Can you work these out from the drawing? Everything is in mm from the part's minimum corner. A direction names the side the tool comes from. Coordinates: 2 decimals unless noted, no trailing zeros. Write each loop counter-clockwise with the first axis right and the second up, starting at its lowest first coordinate (ties: lowest second). Pieces come first, ordered by that corner, then holes. Notation, with made-up numbers: M 86.5,29 L 133.5,29 A14 ccw 133.5,45 Z; hole C -28,30.5 d4. An arc over 180 degrees is marked long. Write item = value, one per line.
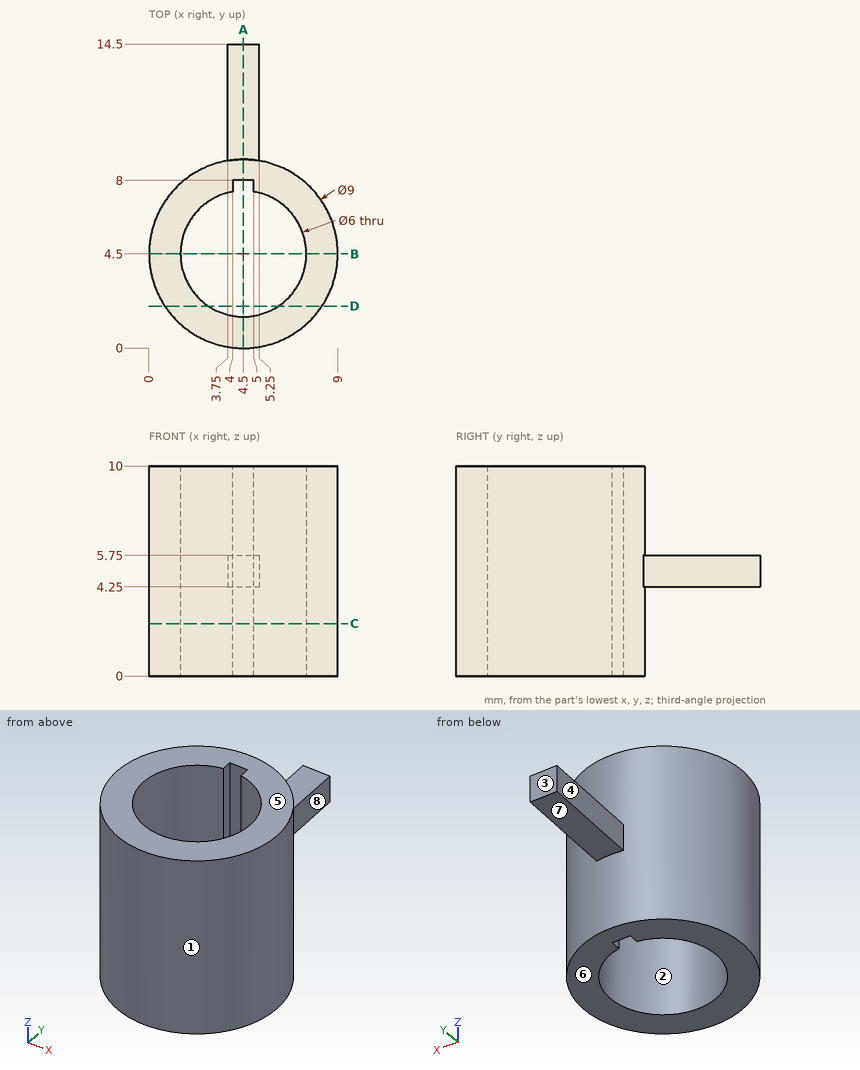
Item 1: For the marked faces 4, 5, 6, 7 and 8, which set-ups out of +Z, -Z, +X, -X, +Y, -Y let a thin tool reach every point of the face, with its end or its side?
Numbers:
face_4 = +Z, -Z, -X, +Y
face_5 = +Z, +X, -X, +Y, -Y
face_6 = -Z, +X, -X, +Y, -Y
face_7 = -Z, +X, -X, +Y
face_8 = +Z, -Z, +X, +Y
Item 2: I'm going to push flat-ended pins straight in: P1, Ø1, axis at y = 10, z = 5, coming from the +X side; P2, Ø1.6, axis at x = 4.5, y = 11.5, coming from the +Z side; P3, Ø6, axis at y = 12, z = 4.5, coming from the -X side. Where does each tip first touch, or does it pass through?
Numbers:
P1 = 5.25
P2 = 5.75
P3 = 3.75
Item 3: Imagine slicing it at D-D (y = 2). Write out the boundary of the cut face in (x, z).
Numbers:
outline = M 0.76,0 L 2.84,0 L 2.84,10 L 0.76,10 Z; M 6.16,0 L 8.24,0 L 8.24,10 L 6.16,10 Z
Item 4: Imagine slicing it at C-C (z = 2.5). Write out the boundary of the cut face in (x, y).
Numbers:
outline = C 4.5,4.5 d9; hole M 4,7.46 A3 ccw long 5,7.46 L 5,8 L 4,8 Z
Item 5: Imagine slicing it at B-B (y = 4.5). Write out the boundary of the cut face in (x, z), and give its area (3 significant figures).
Numbers:
outline = M 0,0 L 1.5,0 L 1.5,10 L 0,10 Z; M 7.5,0 L 9,0 L 9,10 L 7.5,10 Z
area = 30.0 mm²
Item 6: Imagine slicing it at A-A (x = 4.5). Write out the boundary of the cut face in (y, z).
Numbers:
outline = M 0,0 L 1.5,0 L 1.5,10 L 0,10 Z; M 8,0 L 9,0 L 9,4.25 L 14.5,4.25 L 14.5,5.75 L 9,5.75 L 9,10 L 8,10 Z
Item 7: If I drill on line 1 along Y through (x, z) = (4.5, 4); line 2 along X through (y, z) = (7.5, 2); line 3 along X through (y, z) = (10, 4.5), over which ranges is the centre line in solid material (lowest first)?
Numbers:
line_1 = 0 to 1.5, 8 to 9
line_2 = 1.15 to 4, 5 to 7.85
line_3 = 3.75 to 5.25
Item 8: If we mould it in two halves opening along X, with no side actions, what happens to the marked faces 1, 2 and 3? For each: pulls with the +X half, pulls with the -X half, needs draft (parallel to the pull), parting line crosses it, or undercut.
Numbers:
face_1 = parting line crosses it
face_2 = undercut
face_3 = needs draft
